Autodesk Inventor part; units mm, degrees
ref_plane "YZ Plane" through (0, 0, 0) normal (1, 0, 0) x (0, 1, 0)
ref_plane "XZ Plane" through (0, 0, 0) normal (0, 1, 0) x (-1, 0, 0)
ref_plane "XY Plane" through (0, 0, 0) normal (0, 0, 1) x (1, 0, 0)
sketch "Sketch1" plane through (0, 0, 0) normal (0, 0, 1) x (1, 0, 0)
  circle A0 centre (0, 0) radius 2
  dimension "d0" = 4
extrude "Extrusion1" add sketch "Sketch1" along normal blind 10.8 and the other way blind 3.2
sketch "Sketch2" plane through (0, 0, 10.8) normal (0, 0, 1) x (1, 0, 0)
  circle A0 centre (0, 0) radius 1.9
  dimension "d3" = 3.8
extrude "Extrusion2" add sketch "Sketch2" along normal blind 0.5
sketch "Sketch3" plane through (0, 0, 11.3) normal (0, 0, 1) x (1, 0, 0)
  circle A0 centre (0, 0) radius 2
extrude "Extrusion3" add sketch "Sketch3" along normal blind 1.65
chamfer "Chamfer1" distance 0.5 angle 45 1 edges at (-2, 0, 12.95)
properties part number "KURBELZAPFEN NEW" material "Steel ASTM A36"
For this review, take the finished solid that the model builds, in its own axes (mm). Round coordinates to 2 decimals unless told otherwise and drop trailing zeros. Write each loop counter-clockwise with the first axis right and the second up, starting at its lowest first coordinate (ties: lowest second). Pieces come first, ordered by that corner, then holes. Notation, with made-up numbers: (81.5, 19) -> (118.5, 19) arc R26 cw to (118.5, 46) -> close; hole circle Ø11 at (33.25, 46). An arc over 180 degrees is marked (long way). One line per question, with ' | ' between items. Start each with the question number.
(1) Add section A-A, the plane z = 10. Write out the cut boundary in (x, y), plus the area to 3 significant figures.
(2) Insertion check: P1, Ø1, axis at x = 1, z = 4.5, coming from the -Y side. The pin has a flat end and moves straight along its axis. Give the tip position at first contact, or say it passes through.
(3) For line 1 along X through (y, z) = (0.1, 9.75); line 2 along X through (y, z) = (0.9, 5), list the stretches that pass through material, from the lowest coordinate up. Write a range as from..to.
(4) Mouldability with a two-part tool opening along Z and no side actions: class faces 1 (the face through (-1.9, -0.08, 11.05)), 2 (the face through (0, -2, 4)), 3 (the face through (0, 0, -3.2)) as released by +Z, released by -Z, zero draft, split by the parting line, or undercut.
Answer list:
1) outline: circle Ø4 at (0, 0) | area: 12.6 mm²
2) P1: y = -1.94
3) line 1: -2..2 | line 2: -1.79..1.79
4) face 1: undercut | face 2: zero draft | face 3: released by -Z
